```python
from build123d import *

# Parameters (mm, degrees)
SKETCH1_W               = 100
SKETCH1_H               = 126
BOSS_EXTRUDE1_DEPTH     = 2
SKETCH2_W               = 96
SKETCH2_H               = 2
BOSS_EXTRUDE2_DEPTH     = 42
CHAMFER1_SIZE           = 32
CHAMFER2_SIZE           = 4
CUT_EXTRUDE1_DEPTH      = 166.577776287
CUT_EXTRUDE1_DEPTH_BACK = 166.577776287
SKETCH4_R               = 11.25
SKETCH4_R_2             = 1.6
SKETCH5_R               = 1.4
SKETCH5_W               = 78
SKETCH5_H               = 28
CUT_EXTRUDE2_DEPTH      = 167.252819525
SKETCH6_W               = 96
SKETCH6_H               = 2
BOSS_EXTRUDE3_DEPTH     = 10
SKETCH9_W               = 4
SKETCH9_H               = 4
SKETCH9_W_2             = 3
BOSS_EXTRUDE5_DEPTH     = 42
SKETCH10_R              = 1.4
CUT_EXTRUDE4_DEPTH      = 10
SKETCH11_W              = 30
SKETCH11_H              = 2
SKETCH11_W_2            = 20
CUT_EXTRUDE5_DEPTH      = 20
CHAMFER4_SIZE           = 2
SKETCH12_R              = 5.5
SKETCH12_R_2            = 7.5
CUT_EXTRUDE6_DEPTH      = 2
SKETCH13_W              = 1
SKETCH13_H              = 10
BOSS_EXTRUDE6_DEPTH     = 12
CHAMFER5_SIZE           = 10
SKETCH14_R              = 1.25
CUT_EXTRUDE7_DEPTH      = 2.3


with BuildPart() as part:
    # Sketch1 → Boss-Extrude1 (new body)
    with BuildSketch(Plane(origin=(0, 0, 0), x_dir=(1, 0, 0), z_dir=(0, 1, 0))):
        with Locations((50, 63)):
            Rectangle(SKETCH1_W, SKETCH1_H)
    extrude(amount=BOSS_EXTRUDE1_DEPTH)

    # Sketch2 → Boss-Extrude2 (add)
    with BuildSketch(Plane(origin=(0, 2, 0), x_dir=(1, 0, 0), z_dir=(0, 1, 0))):
        Polygon((0, 126), (0, 0), (2, 0), (2, 44), (2, 46), (2, 76), (2, 78), (2, 124), (98, 124), (98, 78), (98, 76), (98, 46), (98, 44), (98, 0), (100, 0), (100, 126), align=None)
        with Locations((50, 77)):
            Rectangle(SKETCH2_W, SKETCH2_H)
        with Locations((50, 45)):
            Rectangle(SKETCH2_W, SKETCH2_H)
    extrude(amount=BOSS_EXTRUDE2_DEPTH)

    # Chamfer1
    chamfer1_edges = [part.edges().sort_by_distance(p)[0] for p in [
        (99, 44, 0),
        (1, 44, 0),
    ]]
    chamfer(chamfer1_edges, length=CHAMFER1_SIZE)

    # Chamfer2
    chamfer2_edges = [part.edges().sort_by_distance(p)[0] for p in [
        (2, 23, -124),
        (98, 23, -124),
        (0, 22, -126),
        (100, 22, -126),
    ]]
    chamfer(chamfer2_edges, length=CHAMFER2_SIZE)

    # Sketch4 → Cut-Extrude1 (cut, two sides: drawn at the far end of the back side and taken through both)
    with BuildSketch(Plane(origin=(2, 0, 0), x_dir=(0, 0, -1), z_dir=(1, 0, 0)).offset(-CUT_EXTRUDE1_DEPTH_BACK)):
        with Locations((99, 23)):
            Circle(SKETCH4_R)
        with Locations((83.5, 38.5)):
            Circle(SKETCH4_R_2)
        with Locations((114.5, 38.5)):
            Circle(SKETCH4_R_2)
        with Locations((114.5, 7.5)):
            Circle(SKETCH4_R_2)
        with Locations((83.5, 7.5)):
            Circle(SKETCH4_R_2)
    extrude(amount=CUT_EXTRUDE1_DEPTH + CUT_EXTRUDE1_DEPTH_BACK, mode=Mode.SUBTRACT)

    # Sketch5 → Cut-Extrude2 (cut, through all)
    with BuildSketch(Plane(origin=(0, 2, 0), x_dir=(1, 0, 0), z_dir=(0, 1, 0))):
        with Locations(Location((8, 70, 0), (0, 0, 270))):
            Circle(SKETCH5_R)
        with Locations(Location((8, 52, 0), (0, 0, 270))):
            Circle(SKETCH5_R)
        with Locations(Location((92, 70, 0), (0, 0, 270))):
            Circle(SKETCH5_R)
        with Locations(Location((92, 52, 0), (0, 0, 270))):
            Circle(SKETCH5_R)
        with Locations((50, 61)):
            Rectangle(SKETCH5_W, SKETCH5_H)
    extrude(amount=-CUT_EXTRUDE2_DEPTH, mode=Mode.SUBTRACT)

    # Sketch6 → Boss-Extrude3 (add)
    with BuildSketch(Plane(origin=(0, 2, 0), x_dir=(1, 0, 0), z_dir=(0, 1, 0))):
        with Locations((50, 1)):
            Rectangle(SKETCH6_W, SKETCH6_H)
    extrude(amount=BOSS_EXTRUDE3_DEPTH)

    # Sketch9 → Boss-Extrude5 (add)
    with BuildSketch(Plane(origin=(0, 2, 0), x_dir=(1, 0, 0), z_dir=(0, 1, 0))):
        with Locations((8, 122)):
            Rectangle(SKETCH9_W, SKETCH9_H)
        with Locations((92, 122)):
            Rectangle(SKETCH9_W, SKETCH9_H)
        with Locations((96.5, 48)):
            Rectangle(SKETCH9_W_2, SKETCH9_H)
        with Locations((3.5, 48)):
            Rectangle(SKETCH9_W_2, SKETCH9_H)
    extrude(amount=BOSS_EXTRUDE5_DEPTH)

    # Sketch10 → Cut-Extrude4 (cut)
    with BuildSketch(Plane(origin=(0, 44, 0), x_dir=(1, 0, 0), z_dir=(0, 1, 0))):
        with Locations(Location((3, 48, 0), (0, 0, 270))):
            Circle(SKETCH10_R)
        with Locations(Location((97, 48, 0), (0, 0, 270))):
            Circle(SKETCH10_R)
        with Locations(Location((92, 122, 0), (0, 0, 270))):
            Circle(SKETCH10_R)
        with Locations(Location((8, 122, 0), (0, 0, 270))):
            Circle(SKETCH10_R)
    extrude(amount=-CUT_EXTRUDE4_DEPTH, mode=Mode.SUBTRACT)

    # Sketch11 → Cut-Extrude5 (cut)
    with BuildSketch(Plane(origin=(0, 44, 0), x_dir=(1, 0, 0), z_dir=(0, 1, 0))):
        with Locations((80, 45)):
            Rectangle(SKETCH11_W, SKETCH11_H)
        with Locations((20, 45)):
            Rectangle(SKETCH11_W, SKETCH11_H)
        with Locations((51, 77)):
            Rectangle(SKETCH11_W_2, SKETCH11_H)
    extrude(amount=-CUT_EXTRUDE5_DEPTH, mode=Mode.SUBTRACT)

    # Chamfer4
    chamfer4_edges = [part.edges().sort_by_distance(p)[0] for p in [
        (41, 24, -77),
        (61, 24, -77),
        (95, 24, -45),
        (65, 24, -45),
        (5, 24, -45),
        (35, 24, -45),
    ]]
    chamfer(chamfer4_edges, length=CHAMFER4_SIZE)

    # Sketch12 → Cut-Extrude6 (cut)
    with BuildSketch(Plane(origin=(0, 0, -126), x_dir=(-1, 0, 0), z_dir=(0, 0, -1))):
        with Locations((-50, 14)):
            Circle(SKETCH12_R)
        with Locations((-50, 30)):
            Circle(SKETCH12_R_2)
    extrude(amount=-CUT_EXTRUDE6_DEPTH, mode=Mode.SUBTRACT)

    # Sketch13 → Boss-Extrude6 (add)
    with BuildSketch(Plane.XY):
        Polygon((51, 2), (50, 2), (50, 0), (59.5, 0), (59.5, 2), align=None)
        Polygon((50, 0), (50, 2), (49, 2), (40.5, 2), (40.5, 0), align=None)
        with Locations((50.5, 7)):
            Rectangle(SKETCH13_W, SKETCH13_H)
        with Locations((49.5, 7)):
            Rectangle(SKETCH13_W, SKETCH13_H)
    extrude(amount=BOSS_EXTRUDE6_DEPTH)

    # Chamfer5
    chamfer5_edges = [part.edges().sort_by_distance(p)[0] for p in [
        (50, 12, 12),
    ]]
    chamfer(chamfer5_edges, length=CHAMFER5_SIZE)

    # Sketch14 → Cut-Extrude7 (cut)
    with BuildSketch(Plane.XZ):
        with BuildLine():
            ThreePointArc((40.5, 6), (40.834936491, 7.25), (41.75, 8.165063509))
            Line((41.75, 8.165063509), (47, 11.196152423))
            ThreePointArc((47, 11.196152423), (48.447085729, 11.795554958), (50, 12))
            Line((50, 12), (40.5, 12))
            Line((40.5, 12), (40.5, 6))
        make_face()
        with BuildLine():
            Line((59.5, 12), (50, 12))
            ThreePointArc((50, 12), (51.552914271, 11.795554958), (53, 11.196152423))
            Line((53, 11.196152423), (58.25, 8.165063509))
            ThreePointArc((58.25, 8.165063509), (59.165063509, 7.25), (59.5, 6))
            Line((59.5, 6), (59.5, 12))
        make_face()
        with Locations(Location((57, 6, 0), (0, 0, 270))):
            Circle(SKETCH14_R)
        with Locations(Location((43, 6, 0), (0, 0, 270))):
            Circle(SKETCH14_R)
    extrude(amount=-CUT_EXTRUDE7_DEPTH, mode=Mode.SUBTRACT)


solid = part.part
```
The listing builds one solid part. Answer for the finished solid, in the listing's coordinates (mm). A direction names the side the tool comes from. Coordinates: 2 decimals unless noted, no trailing zeros. Order: outer loops, then holes, each group sorted by start corner. A loop starts at its lowest first (then second) coordinate and runs counter-clockwise, first axis right, second up. Notation, with made-up numbers: M -20,8.25 L 1,8.25 A22 cw 1,26.25 Z; hole C 19.25,89.5 d3. An arc over 180 degrees is marked long. Answer as a JSON object with one key per item and string values. Group by question number.
1. Section A-A on z = -83.5 is taken. Write down the section's boundary in (x, y).
2. Flat-ended cylindrical pins translate along their axes: P1, Ø12, axis at y = 9.5, z = -5, coming from the -X side; P2, Ø4, axis at x = 20.5, y = 20.5, coming from the +Z side; P3, Ø3, axis at y = 5.5, z = 5.5, coming from the +X side; P4, Ø20, axis at y = 23, z = -99, coming from the -X side. Find the tip coordinate at first contact, or state that the pin passes through.
3. Straight lines are drawn through the part: line 1 (Y direction, x = 1.3, z = -114.5); line 2 (X direction, y = 38, z = -122); line 3 (X direction, y = 27, z = -69). For each, find the intervals that lie inside material, in ascending order.
4. A tool of negligible diameter and unlimited length cuts with its end or side. For faces 4 (the flat face through (55, 2, 5)), 5 (the flat face through (98, 23, -63)), 6 (the cylindrical face through (0.99, 18.69, -109.39)), from which of +Z, -Z, +X, -X, +Y, -Y can it reach the whole face along a straight path? Write none if from no direction.
5. Section C-C on y = 14 is taken. State how many separate pieces and enclosed holes the cut face has, then the cut area to 3 significant figures.
6. Section B-B on z = -99 is taken. Write down the section's boundary in (x, y).
7. Determine the mould class of faces 1 (the flat face through (10, 23, -122)), 2 (the cylindrical face through (46.539, 23.346, -125.014)), 3 (the flat face through (99, 28, -16)) for opening direction Z: released by +Z, released by -Z, zero draft, split by the parting line, or undercut.
8. Section D-D on x = 38 is taken. Write down the section's boundary in (y, z).
Values follow:
{
 "1": {"outline": "M 0,0 L 100,0 L 100,5.9 L 98,5.9 L 98,2 L 2,2 L 2,5.9 L 0,5.9 Z; M 0,9.1 L 2,9.1 L 2,36.9 L 0,36.9 Z; M 0,40.1 L 2,40.1 L 2,44 L 0,44 Z; M 98,9.1 L 100,9.1 L 100,36.9 L 98,36.9 Z; M 98,40.1 L 100,40.1 L 100,44 L 98,44 Z"},
 "2": {"P1": "x = 0", "P2": "z = -44", "P3": "x = 51", "P4": "through"},
 "3": {"line 1": "0 to 5.9, 9.1 to 36.9, 40.1 to 44", "line 2": "0 to 4, 6 to 6.6, 9.4 to 10, 90 to 90.6, 93.4 to 94, 96 to 100", "line 3": "0 to 2, 98 to 100"},
 "4": {"face 4": "+Z, +X, +Y", "face 5": "+Y", "face 6": "+X, -X"},
 "5": {"separate pieces": "3", "enclosed holes": "1", "area": "1,050 mm2"},
 "6": {"outline": "M 0,0 L 100,0 L 100,11.75 L 98,11.75 L 98,2 L 2,2 L 2,11.75 L 0,11.75 Z; M 0,34.25 L 2,34.25 L 2,44 L 0,44 Z; M 98,34.25 L 100,34.25 L 100,44 L 98,44 Z"},
 "7": {"face 1": "undercut", "face 2": "zero draft", "face 3": "released by +Z"},
 "8": {"outline": "M 0,-126 L 44,-126 L 44,-124 L 2,-124 L 2,-78 L 44,-78 L 44,-76 L 2,-76 L 2,-75 L 0,-75 Z; M 0,-47 L 2,-47 L 2,-46 L 44,-46 L 44,-44 L 2,-44 L 2,-2 L 12,-2 L 12,0 L 0,0 Z"}
}
